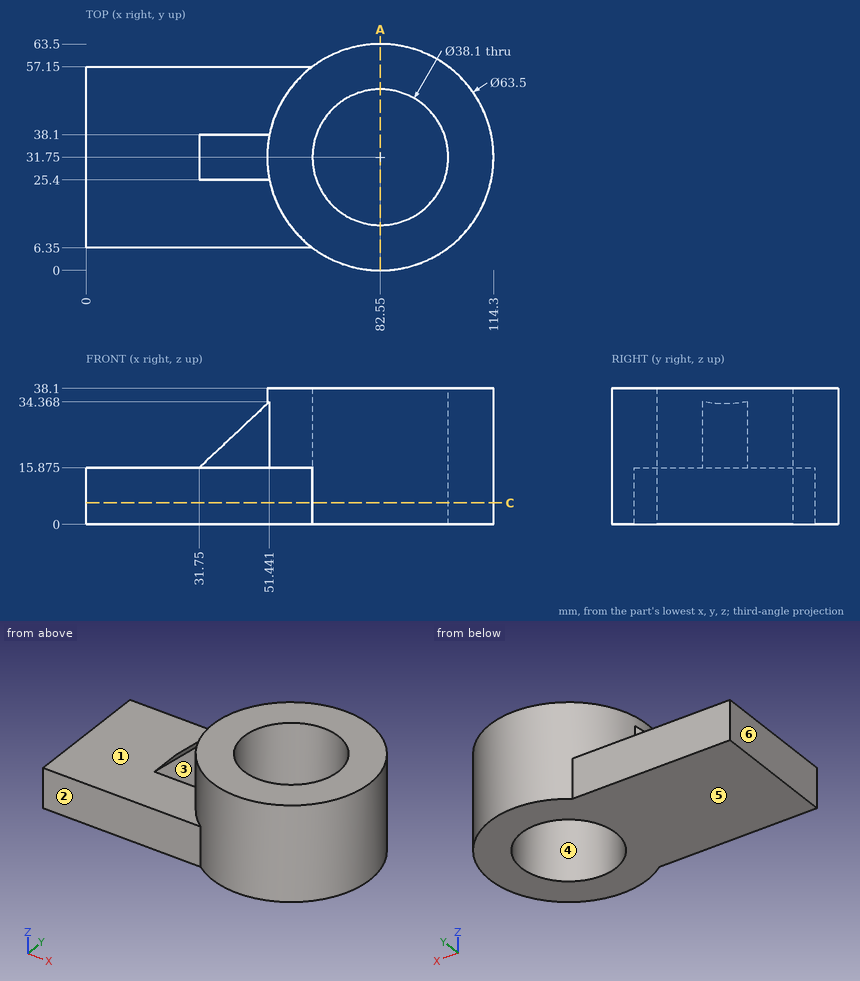
For this review, use the dimensioned drawing (mm, ordinates from the lowest corner) and the shaded views. A direction names the side the tool comes from. Coordinates: 2 decimals unless noted, no trailing zeros. Loops run counter-clockwise (first coordinate to the right, second up) from the corner with the lowest first, then second, coordinate; pieces in that order, holes last. Notation, with made-up numbers: (54, -8) -> (67, -8) arc R16 cw to (67, 19) -> close; hole circle Ø8 at (-35, 78.5). An arc over 180 degrees is marked (long way). Use a Markdown table: item, result. Add a question column.
Item 1: Wall thickness on L1, parallel to X at y = 31, z = 9 (1 decimal); L2, parallel to Y at x = 82, z = 20 (1 decimal); L3, parallel to X at y = 37.5, z = 30 (1 decimal): over which ranges is each line inside the solid? List them lowest first. Write a range as from..to.
Item 2: Machinability: for the marked faces 1, 2 and 3, which of the approach directions +Z, -Z, +X, -X, +Y, -Y give a long, thin tool a straight path to every point of the face, cutting with its end or side? Answer none if there is none.
Item 3: We need section C-C, the plane z = 6. Write out the cut boundary in (x, y).
Item 4: Clearance check with flat-ended pins moving along their axes: P1, Ø20.5, axis at x = 43, z = 24.5, coming from the +Y side; P2, Ø9, axis at x = 40, z = 24.5, coming from the -Y side; P3, Ø8, axis at x = 32, z = 11.5, coming from the -Y side. State where each tip first meets the part, or that it passes through.
Item 5: We need section A-A, the plane x = 82.55. Write out the cut boundary in (y, z), and give its area (3 significant figures).
Item 6: The part is to be moulded in two halves that separate along X. For the marked faces 4, 5 and 6, say which applies: +X half, -X half, draft (parallel to the pull), parting line (faces both ways), or undercut.
Numbers:
| question | item | result |
|---|---|---|
| 1 | L1 | x = 0..63.5, 101.6..114.3 |
| 1 | L2 | y = 0..12.7, 50.8..63.5 |
| 1 | L3 | x = 46.8..64.4, 100.7..113.8 |
| 2 | face 1 | +Z, -X |
| 2 | face 2 | +Z, -Z, -X, -Y |
| 2 | face 3 | +Z, -X, -Y |
| 3 | outline | (0, 6.35) -> (63.5, 6.35) arc R31.75 ccw (long way) to (63.5, 57.15) -> (0, 57.15) -> close; hole circle Ø38.1 at (82.55, 31.75) |
| 4 | P1 | stops at y = 57.15 |
| 4 | P2 | stops at y = 25.4 |
| 4 | P3 | stops at y = 6.35 |
| 5 | outline | (0, 0) -> (12.7, 0) -> (12.7, 38.1) -> (0, 38.1) -> close; (50.8, 0) -> (63.5, 0) -> (63.5, 38.1) -> (50.8, 38.1) -> close |
| 5 | area | 968 mm^2 |
| 6 | face 4 | undercut |
| 6 | face 5 | draft |
| 6 | face 6 | -X half |
